Check sheet for the modelled part. Datum: model origin and axes. Units: mm. A direction names the side the tool comes from. Round coordinates to 2 decimals unless told otherwise and drop trailing zeros. Write each loop counter-clockwise with the first axis right and the second up, starting at its lowest first coordinate (ties: lowest second). Pieces come first, ordered by that corner, then holes. Notation, with made-up numbers: (76, 2.5) -> (83, 2.5) arc R36 cw to (83, 40.5) -> close; hole circle Ø5 at (62.25, 65.5). An arc over 180 degrees is marked (long way). Put each result on its own line as item: value. Start each with the question number.
from build123d import *

# Parameters (mm, degrees)
F1_DEPTH      = 60
F3_DEPTH      = 86.6164273188
F3_DEPTH_BACK = 86.6164273188
F5_DEPTH      = 8.001


with BuildPart() as f1:
    # F0 (on Front) → F1 (new body)
    with BuildSketch(Plane.XZ):
        with BuildLine():
            ThreePointArc((-66.4719767662, 14.8236190979), (-59.3286888206, 4.1329331942), (-47.1534602404, 0))
            Line((-47.1534602404, 0), (47.1534602404, 0))
            ThreePointArc((47.1534602404, 0), (59.3286888206, 4.1329331942), (66.4719767662, 14.8236190979))
            Line((66.4719767662, 14.8236190979), (86.6154273188, 90))
            Line((86.6154273188, 90), (78.8880207085, 92.0705523608))
            Line((78.8880207085, 92.0705523608), (58.7445701559, 16.8941714588))
            ThreePointArc((58.7445701559, 16.8941714588), (54.4585973885, 10.4797599165), (47.1534602404, 8))
            Line((47.1534602404, 8), (-47.1534602404, 8))
            ThreePointArc((-47.1534602404, 8), (-54.4585973885, 10.4797599165), (-58.7445701559, 16.8941714588))
            Line((-58.7445701559, 16.8941714588), (-78.8880207085, 92.0705523608))
            Line((-78.8880207085, 92.0705523608), (-86.6154273188, 90))
            Line((-86.6154273188, 90), (-66.4719767662, 14.8236190979))
        make_face()
    extrude(amount=F1_DEPTH)

    # F2 (on Right) → F3 (cut, two sides)
    with BuildSketch(Plane.YZ) as f3_sk:
        Polygon((-15, 92.0705523608), (-60, 92.0705523608), (-60, 10), align=None)
    extrude(amount=-F3_DEPTH, mode=Mode.SUBTRACT)
    extrude(f3_sk.sketch, amount=F3_DEPTH_BACK, mode=Mode.SUBTRACT)

    # F4 (on face) → F5 (cut, through all)
    with BuildSketch(Plane.XY.offset(8)):
        with BuildLine():
            Line((-33, -26), (-33, -34))
            ThreePointArc((-33, -34), (-25, -42), (-17, -34))
            Line((-17, -34), (-17, -26))
            ThreePointArc((-17, -26), (-25, -18), (-33, -26))
        make_face()
        with BuildLine():
            ThreePointArc((33, -26), (25, -18), (17, -26))
            Line((17, -26), (17, -34))
            ThreePointArc((17, -34), (25, -42), (33, -34))
            Line((33, -34), (33, -26))
        make_face()
    extrude(amount=-F5_DEPTH, mode=Mode.SUBTRACT)


solid = f1.part
1. Access from +Z, -Z, +X, -X, +Y, -Y to the whole of each face (thin tool, end or side, straight path). Record for faces 1 (the flat face through (66.72, -21.47, 46.66)), 2 (the flat face through (82.81, -7.95, 91.02)), 3 (the cylindrical face through (25, -42, 4)).
2. Gauge pin test, flat ends, axial feed: P1, Ø3, axis at x = -62, y = -11, coming from the -Z side; P2, Ø9, axis at y = -31, z = 2, coming from the +X side; P3, Ø1, axis at y = -20.5, z = 27, coming from the -X side. Record the tip position at first contact, or that the pin passes through.
3. Section check B-B, the plane z = 34.5. Enter the section's corners in (x, y).
4. Section check D-D, the plane y = -37. Enter the section's corners in (x, z), then the cut area to 3 significant figures.
5. Section check C-C, the plane y = -12. Enter the section's corners in (x, z), then the cut area to 3 significant figures.
6. Material ranges on L1, parallel to X at y = -17, z = 88; L2, parallel to X at y = -9, z = 9.5; L3, parallel to Z at x = 16.5, y = -11, recorded low to high. Write a range as [from, to].
7. Draft check along X on faces 4 (the flat face through (-72.556, -37.605, 50.844)), 5 (the cylindrical face through (54.55, -29.58, 10.55)), 6 (the flat face through (74.165, -21.903, 43.533)), 7 (the flat face through (-82.7, -7.95, 91.05)). Enter one of: released by +X, released by -X, zero draft, split by the parting line, or undercut.
8. Section check A-A, the plane x = -25. Enter the section's corners in (y, z).
Reply:
1. face 1: +Z, +Y, -Y
1. face 2: +Z, +X, +Y, -Y
1. face 3: +Z, -Z
2. P1: stops at z = 5.1
2. P2: stops at x = 61.91
2. P3: stops at x = -69.87
3. outline: (-71.74, -46.57) -> (-63.46, -46.57) -> (-63.46, 0) -> (-71.74, 0) -> close; (63.46, -46.57) -> (71.74, -46.57) -> (71.74, 0) -> (63.46, 0) -> close
4. outline: (-76.42, 51.95) -> (-66.47, 14.82) arc R20 ccw to (-47.15, 0) -> (-32.42, 0) -> (-32.42, 8) -> (-47.15, 8) arc R12 cw to (-58.74, 16.89) -> (-68.14, 51.95) -> close; (-17.58, 0) -> (17.58, 0) -> (17.58, 8) -> (-17.58, 8) -> close; (32.42, 0) -> (47.15, 0) arc R20 ccw to (66.47, 14.82) -> (76.42, 51.95) -> (68.14, 51.95) -> (58.74, 16.89) arc R12 cw to (47.15, 8) -> (32.42, 8) -> close
4. area: 1,450 mm2
5. outline: (-86.62, 90) -> (-66.47, 14.82) arc R20 ccw to (-47.15, 0) -> (47.15, 0) arc R20 ccw to (66.47, 14.82) -> (86.62, 90) -> (78.89, 92.07) -> (58.74, 16.89) arc R12 cw to (47.15, 8) -> (-47.15, 8) arc R12 cw to (-58.74, 16.89) -> (-78.89, 92.07) -> close
5. area: 2,330 mm2
6. L1: x = [-86.08, -77.8], [77.8, 86.08]
6. L2: x = [-64.18, -52.96], [52.96, 64.18]
6. L3: z = [0, 8]
7. face 4: zero draft
7. face 5: undercut
7. face 6: released by +X
7. face 7: released by -X
8. outline: (-60, 0) -> (-42, 0) -> (-42, 8) -> (-60, 8) -> close; (-18, 0) -> (0, 0) -> (0, 8) -> (-18, 8) -> close
